```python
from build123d import *

# Parameters (mm, degrees)
SKETCH1_R           = 2.5
BOSS_EXTRUDE1_DEPTH = 24
SKETCH2_W           = 24
SKETCH2_H           = 16
CUT_EXTRUDE1_DEPTH  = 23
CUT_EXTRUDE2_DEPTH  = 6.8
SKETCH6_R           = 4.1
CUT_EXTRUDE3_DEPTH  = 17


with BuildPart() as part:
    # Sketch1 → Boss-Extrude1 (new body)
    with BuildSketch(Plane.XY):
        with BuildLine():
            Line((0, 11), (30, 11))
            Line((30, 11), (30, -11))
            Line((30, -11), (0, -11))
            ThreePointArc((0, -11), (-11, 0), (0, 11))
        make_face()
        Circle(SKETCH1_R, mode=Mode.SUBTRACT)
    extrude(amount=BOSS_EXTRUDE1_DEPTH)

    # Sketch2 → Cut-Extrude1 (cut, through all)
    with BuildSketch(Plane(origin=(0, 11, 0), x_dir=(1, 0, 0), z_dir=(0, 1, 0))):
        with Locations((1, -12)):
            Rectangle(SKETCH2_W, SKETCH2_H)
    extrude(amount=-CUT_EXTRUDE1_DEPTH, mode=Mode.SUBTRACT)

    # Sketch4 → Cut-Extrude2 (cut)
    with BuildSketch(Plane(origin=(26, 0, 0), x_dir=(0, 0, -1), z_dir=(1, 0, 0))):
        Polygon((-18.5, 3.75277675), (-18.5, -11), (-5.5, -11), (-5.5, 3.75277675), (-12, 7.505553499), align=None)
    extrude(amount=-CUT_EXTRUDE2_DEPTH, mode=Mode.SUBTRACT)

    # Sketch6 → Cut-Extrude3 (cut)
    with BuildSketch(Plane(origin=(30, 0, 0), x_dir=(0, 0, -1), z_dir=(1, 0, 0))):
        with Locations((-12, 0)):
            Circle(SKETCH6_R)
    extrude(amount=-CUT_EXTRUDE3_DEPTH, mode=Mode.SUBTRACT)


solid = part.part
```
CAD build for the part. Positions are in the model's coordinates, mm. A direction names the side the tool comes from. Give positions to 0.01 mm unless a question says otherwise; leave off trailing zeros. Loops run counter-clockwise (first coordinate to the right, second up) from the corner with the lowest first, then second, coordinate; pieces in that order, holes last. Notation, with made-up numbers: M -14,56 L 16,56 A15 cw 16,85 Z; hole C -24,77.25 d6. An arc over 180 degrees is marked long. Use one line per item in the form item = value.
Item 1: Slice it at B-B (x = -1.5). List the corners of the cut face in (y, z).
Determined:
outline = M -10.9,0 L -2,0 L -2,4 L -10.9,4 Z; M -10.9,20 L -2,20 L -2,24 L -10.9,24 Z; M 2,0 L 10.9,0 L 10.9,4 L 2,4 Z; M 2,20 L 10.9,20 L 10.9,24 L 2,24 Z
Item 2: Drill centre lines: probe 1 along Z at (x, y) = (9.5, 0.5); probe 2 along X at (y, z) = (6, 11.75); probe 3 along Y at (x, z) = (16.5, 12). Where is each one in solid material? Low to high. Write a range as from..to.
Determined:
probe_1 = 0..4, 20..24
probe_2 = 13..19.2, 26..30
probe_3 = -11..-4.1, 4.1..11
Item 3: Which spindle directions (+Z, -Z, +X, -X, +Y, -Y) get a long thin tool onto all of the face, cutting with end or side? Do faces 5 (the face through (23, -4, 18.5)), 6 (the face through (3, 0, 4)), 7 (the face through (-11, 0, 2)). Say none if no direction does.
Determined:
face_5 = -Y
face_6 = -X, +Y, -Y
face_7 = +Z, -Z, -X
Item 4: Slice it at C-C (x = 18). List the corners of the cut face in (y, z).
Determined:
outline = M -11,0 L 11,0 L 11,24 L -11,24 Z; hole C 0,12 d8.2
Item 5: Slice it at A-A (y = 0). List the corners of the cut face in (x, z).
Determined:
outline = M -11,0 L -2.5,0 L -2.5,4 L -11,4 Z; M -11,20 L -2.5,20 L -2.5,24 L -11,24 Z; M 2.5,0 L 30,0 L 30,7.9 L 26,7.9 L 26,5.5 L 19.2,5.5 L 19.2,7.9 L 13,7.9 L 13,4 L 2.5,4 Z; M 2.5,20 L 13,20 L 13,16.1 L 19.2,16.1 L 19.2,18.5 L 26,18.5 L 26,16.1 L 30,16.1 L 30,24 L 2.5,24 Z
Item 6: Flat gauge pins, fed straight in: pin 1 (2 mm diameter, centred on y = -2.5, z = 4.5, fed in from -X); pin 2 (7.5 mm diameter, centred on y = 0, z = 12, fed in from -X); pin 3 (1 mm diameter, centred on y = 7.5, z = 14.5, fed in from -X). Where does each tip first touch, or does it go through?
Determined:
pin_1 = -10.88
pin_2 = through
pin_3 = 13
Item 7: Slice it at D-D (y = 3.25). List the corners of the cut face in (x, z).
Determined:
outline = M -10.51,0 L 30,0 L 30,9.5 L 26,9.5 L 26,5.5 L 19.2,5.5 L 19.2,9.5 L 13,9.5 L 13,4 L -10.51,4 Z; M -10.51,20 L 13,20 L 13,14.5 L 19.2,14.5 L 19.2,18.5 L 26,18.5 L 26,14.5 L 30,14.5 L 30,24 L -10.51,24 Z
Item 8: Two-plate mould, pull along X, no slides. Class faces 1 (the face through (10, 0, 0)), 2 (the face through (26, -6, 12)), 3 (the face through (22.6, 5.6, 8.7)), 4 (the face through (13, 3, 16)): pulls with the +X half, pulls with the -X half, needs draft (parallel to the pull), parting line crosses it, or undercut.
Determined:
face_1 = needs draft
face_2 = undercut
face_3 = undercut
face_4 = pulls with the -X half
